Geometry: final body of the model. Coordinates: model frame, mm. A direction names the side the tool comes from. Give positions to 0.01 mm unless a question says otherwise; leave off trailing zeros. Loops run counter-clockwise (first coordinate to the right, second up) from the corner with the lowest first, then second, coordinate; pieces in that order, holes last.
from build123d import *

# Parameters (mm, degrees)
SKETCH_W      = 60
SKETCH_H      = 60
PAD_DEPTH     = 6
SKETCH001_R   = 20
SKETCH001_R_2 = 15
PAD001_DEPTH  = 20


with BuildPart() as part:
    # Sketch → Pad (new body)
    with BuildSketch(Plane.XY):
        Rectangle(SKETCH_W, SKETCH_H)
    extrude(amount=-PAD_DEPTH)

    # Sketch001 → Pad001 (join)
    with BuildSketch(Plane.XY):
        Circle(SKETCH001_R)
        Circle(SKETCH001_R_2, mode=Mode.SUBTRACT)
    extrude(amount=PAD001_DEPTH)


solid = part.part
Item 1: Draft query along Y for faces 1 (the face through (-14.985, 0.66, 9.86)), 2 (the face through (-4.336, -19.524, 9.86)), 3 (the face through (0, 0, 0)), 4 (the face through (0, 0, -6)). Return one class per face: +Y half, -Y half, draft (parallel to the pull), parting line (faces both ways), or undercut.
Values follow:
face 1: undercut
face 2: parting line
face 3: undercut
face 4: draft
Item 2: Section query D-D on x = -18. Return loops of the section in (y, z).
Values follow:
outline: (-30, -6) - (30, -6) - (30, 0) - (8.72, 0) - (8.72, 20) - (-8.72, 20) - (-8.72, 0) - (-30, 0) - close
Item 3: Ray query, probe 1 along Y at (x, z) = (0, 10.5); probe 2 along Z at (x, y) = (20.5, 23); probe 3 along Y at (x, z) = (5, 5). Return the intervals inside material, ascending.
Values follow:
probe 1: y = -20 to -15, 15 to 20
probe 2: z = -6 to 0
probe 3: y = -19.36 to -14.14, 14.14 to 19.36
Item 4: Section query C-C on z = 2.75. Return loops of the section in (x, y).
Values follow:
outline: circle Ø40 at (0, 0); hole circle Ø30 at (0, 0)
Item 5: Section query A-A on x = 0. Return loops of the section in (y, z).
Values follow:
outline: (-30, -6) - (30, -6) - (30, 0) - (20, 0) - (20, 20) - (15, 20) - (15, 0) - (-15, 0) - (-15, 20) - (-20, 20) - (-20, 0) - (-30, 0) - close
Item 6: Pin query (flat end, axial travel): pin 1 (8 mm diameter, centred on x = -8.5, z = 11, fed in from +Y); pin 2 (12 mm diameter, centred on x = 18.5, z = 11, fed in from -Y); pin 3 (4 mm diameter, centred on x = 5, z = 1.5, fed in from -Y); pin 4 (15 mm diameter, centred on x = -4.5, y = -3, fed in from +Z). Return the tip coordinate at first contact, or that it passes through.
Values follow:
pin 1: stops at y = 19.49
pin 2: stops at y = -15.61
pin 3: stops at y = -30
pin 4: stops at z = 0
Item 7: Set-up query: faces 5 (the face through (-30, 0, -3)), 6 (the face through (-0.4, 20.4, 0)). Return all of +Z, -Z, +X, -X, +Y, -Y with unobstructed straight access to the full face (end or side cutting, diameter ignored); none if empty.
Values follow:
face 5: +Z, -Z, -X, +Y, -Y
face 6: +Z
